Check sheet for the modelled part. Datum: model origin and axes. Units: mm. A direction names the side the tool comes from. Round coordinates to 2 decimals unless told otherwise and drop trailing zeros. Loops run counter-clockwise (first coordinate to the right, second up) from the corner with the lowest first, then second, coordinate; pieces in that order, holes last. Notation, with made-up numbers: (3.25, -13) -> (25.25, -13) arc R20 ccw to (25.25, 13) -> close; hole circle Ø1 at (-10, -32.75). An arc over 180 degrees is marked (long way). Return JSON: item names as keys, results as strings.
from build123d import *

# Parameters (mm, degrees)
SKETCH_1_W          = 42
SKETCH_1_H          = 42
EXTRUDE_1_DEPTH     = 48
SKETCH_2_R          = 11
EXTRUDE_2_DEPTH     = 2
SKETCH_3_R          = 2.25
EXTRUDE_3_DEPTH     = 22
SKETCH_4_R          = 1.5
CUT_EXTRUDE_1_DEPTH = 4.5
FILLET_1_R          = 5
SKETCH_5_R          = 2.5
EXTRUDE_4_DEPTH     = 20


with BuildPart() as part:
    # 草图1 → 凸台-拉伸1 (new body)
    with BuildSketch(Plane.XY):
        Rectangle(SKETCH_1_W, SKETCH_1_H)
    extrude(amount=EXTRUDE_1_DEPTH)

    # 草图2 → 凸台-拉伸2 (add)
    with BuildSketch(Plane(origin=(0, 0, 0), x_dir=(-1, 0, 0), z_dir=(0, 0, -1))):
        Circle(SKETCH_2_R)
    extrude(amount=EXTRUDE_2_DEPTH)

    # 草图3 → 凸台-拉伸3 (add)
    with BuildSketch(Plane(origin=(0, 0, -2), x_dir=(-1, 0, 0), z_dir=(0, 0, -1))):
        Circle(SKETCH_3_R)
    extrude(amount=EXTRUDE_3_DEPTH)

    # 草图4 → 切除-拉伸1 (cut)
    with BuildSketch(Plane(origin=(0, 0, 0), x_dir=(-1, 0, 0), z_dir=(0, 0, -1))):
        with Locations((-15.5, 15.5)):
            Circle(SKETCH_4_R)
        with Locations((15.5, 15.5)):
            Circle(SKETCH_4_R)
        with Locations((15.5, -15.5)):
            Circle(SKETCH_4_R)
        with Locations((-15.5, -15.5)):
            Circle(SKETCH_4_R)
    extrude(amount=-CUT_EXTRUDE_1_DEPTH, mode=Mode.SUBTRACT)

    # 圆角1
    fillet_1_edges = [part.edges().sort_by_distance(p)[0] for p in [
        (21, -21, 24),
        (-21, -21, 24),
        (-21, 21, 24),
        (21, 21, 24),
    ]]
    fillet(fillet_1_edges, radius=FILLET_1_R)

    # 草图5 → 凸台-拉伸4 (add)
    with BuildSketch(Plane.XY.offset(48)):
        Circle(SKETCH_5_R)
    extrude(amount=EXTRUDE_4_DEPTH)


solid = part.part
Q1. Go/stop test with flat-tipped pins: pin 1 (3.5 mm diameter, centred on x = 16, y = -15, fed in from -Z); pin 2 (4 mm diameter, centred on x = 15.5, y = -15.5, fed in from +Z); pin 3 (1 mm diameter, centred on x = -4.5, y = 5, fed in from -Z); pin 4 (5 mm diameter, centred on x = -5, z = -8, fed in from +Y). Record where each tip stops, or that it passes through.
Results list:
{"pin 1": "z = 0", "pin 2": "z = 48", "pin 3": "z = -2", "pin 4": "through"}
Q2. Section check A-A (x = 0). Record the boundary of the cut face in (y, z), then the cut area to 3 significant figures.
Results list:
{"outline": "(-21, 0) -> (-11, 0) -> (-11, -2) -> (-2.25, -2) -> (-2.25, -24) -> (2.25, -24) -> (2.25, -2) -> (11, -2) -> (11, 0) -> (21, 0) -> (21, 48) -> (2.5, 48) -> (2.5, 68) -> (-2.5, 68) -> (-2.5, 48) -> (-21, 48) -> close", "area": "2,260 mm^2"}
Q3. Section check C-C (z = -3.5). Record the boundary of the cut face in (x, y).
Results list:
{"outline": "circle Ø4.5 at (0, 0)"}
Q4. Tool access check on faces 1 (the flat face through (0, 0, 68)), 2 (the cylindrical face through (-0.54, -2.44, 57.86)), 3 (the cylindrical face through (2.38, -10.74, -0.99)). Record the directions out of +Z, -Z, +X, -X, +Y, -Y that give a thin tool (end or side, any length) a straight path to the whole face; none if there is none.
Results list:
{"face 1": "+Z, +X, -X, +Y, -Y", "face 2": "+Z", "face 3": "-Z"}
Q5. Material ranges on line 1 (Y direction, x = 15.5, z = 1.35); line 2 (Y direction, x = -15, z = 3); line 3 (Z direction, x = -8.5, y = -16.5), recorded low to high.
Results list:
{"line 1": "-21 to -17, -14 to 14, 17 to 21", "line 2": "-21 to -16.91, -14.09 to 14.09, 16.91 to 21", "line 3": "0 to 48"}
Q6. Draft check along X on faces 4 (the cylindrical face through (-14, 15.57, 2.22)), 5 (the flat face through (-21, 0, 24)), 6 (the cylindrical face through (-14, -15.43, 2.22)), 7 (the flat face through (21, 0, 24)). Enter one of: released by +X, released by -X, zero draft, split by the parting line, or undercut.
Results list:
{"face 4": "undercut", "face 5": "released by -X", "face 6": "undercut", "face 7": "released by +X"}
Q7. Section check D-D (y = 6). Record the boundary of the cut face in (x, z), then the cut area to 3 significant figures.
Results list:
{"outline": "(-21, 0) -> (-9.22, 0) -> (-9.22, -2) -> (9.22, -2) -> (9.22, 0) -> (21, 0) -> (21, 48) -> (-21, 48) -> close", "area": "2,050 mm^2"}
